```python
from build123d import *
from OCP.BRepFilletAPI import BRepFilletAPI_MakeChamfer

# Parameters (mm, degrees)
EXTRUDE_1_DEPTH                                 = 15.7
CUT_EXTRUDE_5_DEPTH                             = 6
CUT_EXTRUDE_START                               = -4
CUT_EXTRUDE_6_DEPTH                             = 4
CHAMFER_2_SIZE                                  = 2.5
CHAMFER_2_SIZE_2                                = 1.5
CHAMFER_3_SIZE                                  = 2.5
CHAMFER_3_SIZE_2                                = 1.5
CHAMFER_4_SIZE                                  = 2.5
CHAMFER_4_SIZE_2                                = 1.5
CHAMFER_5_SIZE                                  = 1.5
CHAMFER_5_SIZE_2                                = 2.5
CUT_EXTRUDE_7_DEPTH                             = 20
BOSS_EXTRUDE2_DEPTH                             = 15
CSK_FOR_M4_FLAT_HEAD_MACHINE_SCREW1_D           = 4.5
CSK_FOR_M4_FLAT_HEAD_MACHINE_SCREW1_DEPTH       = 28.648063607
CSK_FOR_M4_FLAT_HEAD_MACHINE_SCREW1_CSINK_D     = 9.4
CSK_FOR_M4_FLAT_HEAD_MACHINE_SCREW1_CSINK_ANGLE = 90
CSK_FOR_M4_FLAT_HEAD_MACHINE_SCREW1_TIP         = 1.351936393
BOSS_EXTRUDE3_DEPTH                             = 3
BOSS_EXTRUDE3_DEPTH_BACK                        = 4.283096
CUT_EXTRUDE1_DEPTH                              = 122.536445899
CUT_EXTRUDE2_START                              = -5
CUT_EXTRUDE2_DEPTH                              = 5
CHAMFER1_SIZE                                   = 5
CUT_EXTRUDE3_REACH                              = 94.592
SKETCH9_R                                       = 2


with BuildPart() as part:
    # Эскиз1 → Бобышка-Вытянуть1 (new body)
    with BuildSketch(Plane(origin=(0, 0, 0), x_dir=(1, 0, 0), z_dir=(0, 1, 0))):
        with BuildLine():
            Line((19, -55.842875467), (21.087010541, -30.364203971))
            ThreePointArc((21.087010541, -30.364203971), (28, -24.464466094), (34.912989459, -30.364203971))
            Line((34.912989459, -30.364203971), (37, -55.842875467))
            ThreePointArc((37, -55.842875467), (49.615065571, -70.216351148), (46.614482007, -89.103732671))
            Line((46.614482007, -89.103732671), (48.9, -97.364070254))
            Line((48.9, -97.364070254), (57, -98.864070254))
            Line((57, -98.864070254), (63.5, -89.453874559))
            Line((63.5, -89.453874559), (64.1, -72.464466094))
            Line((64.1, -72.464466094), (56, 0))
            Line((56, 0), (52.464466094, 3.535533906))
            Line((52.464466094, 3.535533906), (43.553055011, 2.275870258))
            Line((43.553055011, 2.275870258), (12.446944989, 2.275870258))
            Line((12.446944989, 2.275870258), (3.535533906, 3.535533906))
            Line((3.535533906, 3.535533906), (0, 0))
            Line((0, 0), (-8.1, -72.464466094))
            Line((-8.1, -72.464466094), (-7.5, -89.453874559))
            Line((-7.5, -89.453874559), (-1, -98.864070254))
            Line((-1, -98.864070254), (7.1, -97.364070254))
            Line((7.1, -97.364070254), (9.385517993, -89.103732671))
            ThreePointArc((9.385517993, -89.103732671), (6.384934429, -70.216351148), (19, -55.842875467))
        make_face()
    extrude(amount=EXTRUDE_1_DEPTH)

    # Эскиз9 → Вырез-Вытянуть5 (cut)
    with BuildSketch(Plane(origin=(0, 15.7, 0), x_dir=(1, 0, 0), z_dir=(0, 1, 0))):
        with BuildLine():
            Line((4.070420212, -98.938601985), (6.67745221, -89.516245887))
            ThreePointArc((6.67745221, -89.516245887), (28, -51.464466094), (49.32254779, -89.516245887))
            Line((49.32254779, -89.516245887), (51.928879153, -98.936069744))
            Line((51.928879153, -98.936069744), (4.070420212, -98.938601985))
        make_face()
    extrude(amount=-CUT_EXTRUDE_5_DEPTH, mode=Mode.SUBTRACT)

    # Эскиз10 → Вырез-Вытянуть6 (cut)
    with BuildSketch(Plane.XZ.offset(CUT_EXTRUDE_START)):
        with BuildLine():
            Line((49.32254779, 89.516245887), (52.714892846, 101.77688678))
            Line((52.714892846, 101.77688678), (2.982429051, 102.870828422))
            Line((2.982429051, 102.870828422), (6.67745221, 89.516245887))
            ThreePointArc((6.67745221, 89.516245887), (28, 51.464466094), (49.32254779, 89.516245887))
        make_face()
    extrude(amount=CUT_EXTRUDE_6_DEPTH, mode=Mode.SUBTRACT)

    # Фаска2
    chamfer_2_edges_1 = [part.edges().sort_by_distance(p)[0] for p in [
        (8.242758997, 9.7, 93.233901463),
    ]]
    chamfer_2_side_1 = [part.faces().sort_by_distance(p)[0] for p in [
        (8.213845332, 9.7, 93.225901463),
    ]]
    chamfer_2_edges_2 = [part.edges().sort_by_distance(p)[0] for p in [
        (6.384934429, 9.7, 70.216351148),
    ]]
    chamfer_2_side_2 = [part.faces().sort_by_distance(p)[0] for p in [
        (6.356114342, 9.7, 70.208020328),
    ]]
    chamfer_2 = BRepFilletAPI_MakeChamfer(part.part.solid().wrapped)
    for e in chamfer_2_edges_1:
        chamfer_2.Add(CHAMFER_2_SIZE - 0.0001, CHAMFER_2_SIZE_2 - 0.0001, e.wrapped, chamfer_2_side_1[0].wrapped)
    for e in chamfer_2_edges_2:
        chamfer_2.Add(CHAMFER_2_SIZE - 0.0001, CHAMFER_2_SIZE_2 - 0.0001, e.wrapped, chamfer_2_side_2[0].wrapped)
    add(Compound.cast(chamfer_2.Shape()), mode=Mode.REPLACE)  # a hair under: the kernel refuses the full size

    # Фаска3
    chamfer_3_edges_1 = [part.edges().sort_by_distance(p)[0] for p in [
        (8.242758997, 4, 93.233901463),
    ]]
    chamfer_3_side_1 = [part.faces().sort_by_distance(p)[0] for p in [
        (8.213845332, 4, 93.225901463),
    ]]
    chamfer_3_edges_2 = [part.edges().sort_by_distance(p)[0] for p in [
        (6.384934429, 4, 70.216351148),
    ]]
    chamfer_3_side_2 = [part.faces().sort_by_distance(p)[0] for p in [
        (6.384934429, 4.03, 70.216351148),
    ]]
    chamfer_3 = BRepFilletAPI_MakeChamfer(part.part.solid().wrapped)
    for e in chamfer_3_edges_1:
        chamfer_3.Add(CHAMFER_3_SIZE - 0.0001, CHAMFER_3_SIZE_2 - 0.0001, e.wrapped, chamfer_3_side_1[0].wrapped)
    for e in chamfer_3_edges_2:
        chamfer_3.Add(CHAMFER_3_SIZE_2 - 0.0001, CHAMFER_3_SIZE - 0.0001, e.wrapped, chamfer_3_side_2[0].wrapped)
    add(Compound.cast(chamfer_3.Shape()), mode=Mode.REPLACE)  # a hair under: the kernel refuses the full size

    # Фаска4
    chamfer_4_edges_1 = [part.edges().sort_by_distance(p)[0] for p in [
        (47.757241003, 9.7, 93.233901463),
    ]]
    chamfer_4_side_1 = [part.faces().sort_by_distance(p)[0] for p in [
        (47.786154668, 9.7, 93.225901463),
    ]]
    chamfer_4_edges_2 = [part.edges().sort_by_distance(p)[0] for p in [
        (49.615065571, 9.7, 70.216351148),
    ]]
    chamfer_4_side_2 = [part.faces().sort_by_distance(p)[0] for p in [
        (49.643885658, 9.7, 70.208020328),
    ]]
    chamfer_4 = BRepFilletAPI_MakeChamfer(part.part.solid().wrapped)
    for e in chamfer_4_edges_1:
        chamfer_4.Add(CHAMFER_4_SIZE - 0.0001, CHAMFER_4_SIZE_2 - 0.0001, e.wrapped, chamfer_4_side_1[0].wrapped)
    for e in chamfer_4_edges_2:
        chamfer_4.Add(CHAMFER_4_SIZE - 0.0001, CHAMFER_4_SIZE_2 - 0.0001, e.wrapped, chamfer_4_side_2[0].wrapped)
    add(Compound.cast(chamfer_4.Shape()), mode=Mode.REPLACE)  # a hair under: the kernel refuses the full size

    # Фаска5
    chamfer_5_edges_1 = [part.edges().sort_by_distance(p)[0] for p in [
        (47.757241003, 4, 93.233901463),
    ]]
    chamfer_5_side_1 = [part.faces().sort_by_distance(p)[0] for p in [
        (47.757241003, 4.03, 93.233901463),
    ]]
    chamfer_5_edges_2 = [part.edges().sort_by_distance(p)[0] for p in [
        (49.615065571, 4, 70.216351148),
    ]]
    chamfer_5_side_2 = [part.faces().sort_by_distance(p)[0] for p in [
        (49.643885658, 4, 70.208020328),
    ]]
    chamfer_5 = BRepFilletAPI_MakeChamfer(part.part.solid().wrapped)
    for e in chamfer_5_edges_1:
        chamfer_5.Add(CHAMFER_5_SIZE - 0.0001, CHAMFER_5_SIZE_2 - 0.0001, e.wrapped, chamfer_5_side_1[0].wrapped)
    for e in chamfer_5_edges_2:
        chamfer_5.Add(CHAMFER_5_SIZE_2 - 0.0001, CHAMFER_5_SIZE - 0.0001, e.wrapped, chamfer_5_side_2[0].wrapped)
    add(Compound.cast(chamfer_5.Shape()), mode=Mode.REPLACE)  # a hair under: the kernel refuses the full size

    # Эскиз11 → Вырез-Вытянуть7 (cut)
    with BuildSketch(Plane(origin=(0, 15.7, 0), x_dir=(1, 0, 0), z_dir=(0, 1, 0))):
        with BuildLine():
            Line((46.426049473, -86.017959352), (46.012822205, -88.379258027))
            add(Edge.make_bspline(
                [(58.862726543, -70.808948625), (60.119619749, -73.228227212), (61.202001727, -77.673197621), (57.883666669, -86.609034293), (49.905997231, -87.608281842), (46.012822205, -88.379258027)],
                knots=[0, 0, 0, 0, 0.305163468, 0.487677304, 1, 1, 1, 1], degree=3))
            ThreePointArc((58.862726543, -70.808948625), (56.072808864, -68.148005462), (57.1, -71.864070254))
            add(Edge.make_bspline(
                [(57.1, -71.864070254), (58.73856603, -74.489449168), (59.890065943, -84.15910166), (49.798382886, -85.957388163), (46.426049473, -86.017959352)],
                knots=[0, 0, 0, 0, 0.454203244, 1, 1, 1, 1], degree=3))
        make_face()
        with BuildLine():
            Line((9.573950527, -86.017959352), (9.987177795, -88.379258027))
            add(Edge.make_bspline(
                [(-2.862726543, -70.808948625), (-4.119619749, -73.228227212), (-5.202001727, -77.673197621), (-1.883666669, -86.609034293), (6.094002769, -87.608281842), (9.987177795, -88.379258027)],
                knots=[0, 0, 0, 0, 0.305163468, 0.487677304, 1, 1, 1, 1], degree=3))
            ThreePointArc((-2.862726543, -70.808948625), (-0.072808864, -68.148005462), (-1.1, -71.864070254))
            add(Edge.make_bspline(
                [(-1.1, -71.864070254), (-2.73856603, -74.489449168), (-3.890065943, -84.15910166), (6.201617114, -85.957388163), (9.573950527, -86.017959352)],
                knots=[0, 0, 0, 0, 0.454203244, 1, 1, 1, 1], degree=3))
        make_face()
    extrude(amount=-CUT_EXTRUDE_7_DEPTH, mode=Mode.SUBTRACT)

    # Sketch5 → Boss-Extrude2 (add)
    with BuildSketch(Plane.XZ):
        Polygon((3.535533906, -3.535533906), (0, 0), (-3.078509959, 27.541059326), (12.727631466, 30.166723248), (28.000118409, 31.014994944), (59.173331778, 28.389357167), (56, 0), (52.464466094, -3.535533906), (43.553055011, -2.275870258), (12.446944989, -2.275870258), align=None)
    extrude(amount=BOSS_EXTRUDE2_DEPTH)

    # CSK for M4 Flat Head Machine Screw1
    with Locations(Plane(origin=(19.370167772, 15.7, 17.779382006), x_dir=(0, 0, 1), z_dir=(0, 1, 0))):
        with Locations((0, 0), (0, 17.26)):
            CounterSinkHole(CSK_FOR_M4_FLAT_HEAD_MACHINE_SCREW1_D / 2, CSK_FOR_M4_FLAT_HEAD_MACHINE_SCREW1_CSINK_D / 2, depth=CSK_FOR_M4_FLAT_HEAD_MACHINE_SCREW1_DEPTH, counter_sink_angle=CSK_FOR_M4_FLAT_HEAD_MACHINE_SCREW1_CSINK_ANGLE)
            with Locations((0, 0, -(CSK_FOR_M4_FLAT_HEAD_MACHINE_SCREW1_DEPTH + CSK_FOR_M4_FLAT_HEAD_MACHINE_SCREW1_TIP / 2))):  # 118° drill point
                Cone(0, CSK_FOR_M4_FLAT_HEAD_MACHINE_SCREW1_D / 2, CSK_FOR_M4_FLAT_HEAD_MACHINE_SCREW1_TIP, mode=Mode.SUBTRACT)

    # Sketch6 → Boss-Extrude3 (add, two sides: drawn at the far end of the back side and taken through both)
    with BuildSketch(Plane.XY.offset(32.6724529).offset(-BOSS_EXTRUDE3_DEPTH_BACK)):
        Polygon((12.822450363, -11.082801181), (12.822450363, 0), (59.173331778, 0), (59.173331778, -15), (39.425133125, -21.709493147), (16.66992259, -21.709493147), align=None)
    extrude(amount=BOSS_EXTRUDE3_DEPTH + BOSS_EXTRUDE3_DEPTH_BACK)

    # Sketch7 → Cut-Extrude1 (cut, through all)
    with BuildSketch(Plane(origin=(59.173331778, 0, 0), x_dir=(0, 0, -1), z_dir=(1, 0, 0))):
        Polygon((-32.6724529, -22.263045792), (-32.6724529, -12.082801181), (-32.6724529, -11.082801181), (-31.6724529, -11.082801181), (-27.1724529, -11.082801181), (-27.1724529, -22.263045792), align=None)
    extrude(amount=-CUT_EXTRUDE1_DEPTH, mode=Mode.SUBTRACT)

    # Sketch8 → Cut-Extrude2 (cut)
    with BuildSketch(Plane(origin=(0, 0, 0), x_dir=(1, 0, 0), z_dir=(0, 1, 0)).offset(CUT_EXTRUDE2_START)):
        with BuildLine():
            Line((35.347799079, -35.6724529), (34.912989459, -30.364203971))
            ThreePointArc((34.912989459, -30.364203971), (28, -24.464466094), (21.087010541, -30.364203971))
            Line((21.087010541, -30.364203971), (20.652200921, -35.6724529))
            Line((20.652200921, -35.6724529), (35.347799079, -35.6724529))
        make_face()
    extrude(amount=CUT_EXTRUDE2_DEPTH, mode=Mode.SUBTRACT)

    # Chamfer1
    chamfer1_edges = [part.edges().sort_by_distance(p)[0] for p in [
        (28, -5, 35.6724529),
    ]]
    chamfer(chamfer1_edges, length=CHAMFER1_SIZE)

    # Sketch9 → Cut-Extrude3 (cut, up to next)
    with BuildSketch(Plane.XY.offset(35.6724529), mode=Mode.PRIVATE) as cut_extrude3_sk1:
        with Locations((28.047527858, -16.709493147)):
            Circle(SKETCH9_R)
    cut_extrude3_tool1 = extrude(cut_extrude3_sk1.sketch, amount=-CUT_EXTRUDE3_REACH, mode=Mode.PRIVATE) & part.part
    add(cut_extrude3_tool1.solids().sort_by_distance((28.047528, -16.709493, 35.672453))[0], mode=Mode.SUBTRACT)


solid = part.part
```
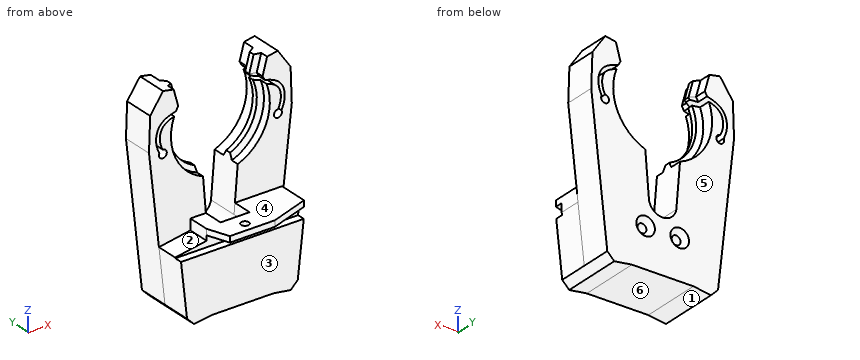
Check sheet for the modelled part. Datum: model origin and axes. Units: mm. Face numbers are marked on the shaded views. A direction names the side the tool comes from. Round coordinates to 2 decimals unless told otherwise and drop trailing zeros. Order: outer loops, then holes, each group sorted by start corner. A loop starts at its lowest first (then second) coordinate and runs counter-clockwise, first axis right, second up.
1) Scan lines: line 1 (Z direction, x = 19, y = -12.5); line 2 (Y direction, x = 38.5, z = 26); line 3 (Y direction, x = 28.5, z = 35). Record each from-to range of solid material in increasing order.
2) Mould release check, pull along X, two halves, no side actions. Record for the marked faces 1, 2 and 3: +X half, -X half, draft (parallel to the pull), parting line (faces both ways), or undercut.
3) Section check A-A (z = 34.5). Record the boundary of the cut face in (x, y).
4) Tool access check on the marked faces 4, 5 and 6. Record the directions out of +Z, -Z, +X, -X, +Y, -Y that give a thin tool (end or side, any length) a straight path to the whole face; none if there is none.
5) Go/stop test with flat-tipped pins: pin 1 Ø1.5 at (x, z) = (17, 41) entering from -Y; pin 2 Ø8 at (y, z) = (-1, 76.5) entering from -X; pin 3 Ø7 at (x, z) = (19.37, 17.78) entering from +Y; pin 4 Ø4 at (x, z) = (21.5, 33.5) entering from +Y. Record where each tip stops, or that it passes through.
6) Section check B-B (z = 82.5). Give the number of separate pieces and of enclosed holes in the cut face, and give its area (3 significant figures).
Result:
1. line 1: z = -2.28 to 15.56, 20 to 27.17, 32.67 to 35.67
1. line 2: y = -15 to 15.7
1. line 3: y = -21.71 to -18.66, -14.76 to -9.33
2. face 1: undercut
2. face 2: -X half
2. face 3: draft
3. outline: (-3.86, 0) - (12.82, 0) - (12.82, -11.08) - (16.67, -21.71) - (39.43, -21.71) - (59.17, -15) - (59.17, 0) - (59.86, 0) - (59.86, 15.7) - (35.25, 15.7) - (35.25, -8.83) - (20.75, -8.83) - (20.75, 15.7) - (-3.86, 15.7) - close; hole circle Ø4 at (28.05, -16.71)
4. face 4: +Z, +X, -X, -Y
4. face 5: +Z, -Z, +X, -X, +Y
4. face 6: -Z, +Y, -Y
5. pin 1: stops at y = 0
5. pin 2: stops at x = -8.09
5. pin 3: stops at y = 14.5
5. pin 4: stops at y = 15.7
6. separate pieces: 4
6. enclosed holes: 0
6. area: 309 mm2
